Check sheet for the modelled part. Datum: model origin and axes. Units: mm. A direction names the side the tool comes from. Coordinates: 2 decimals unless noted, no trailing zeros. Loops run counter-clockwise (first coordinate to the right, second up) from the corner with the lowest first, then second, coordinate; pieces in that order, holes last.
```python
from build123d import *

# Parameters (mm, degrees)
F0_W     = 71.12
F0_H     = 71.12
F1_DEPTH = 43.18
F2_W     = 66.04
F2_H     = 66.04
F3_DEPTH = 40.64
F5_R     = 2.54
F4_W     = 71.12
F4_H     = 71.12
F4_W_2   = 3.81
F4_H_2   = 3.81
F6_DEPTH = 2.54
F7_R     = 2.53999


# Not quite as in the source:
# - a fillet or chamfer is up to 0.001 mm smaller than in the source, because OpenCascade refuses the exact size


with BuildPart() as f1:
    # F0 (on Top) → F1 (new body)
    with BuildSketch(Plane.XY):
        with Locations((35.56, 35.56)):
            Rectangle(F0_W, F0_H)
    extrude(amount=F1_DEPTH)

    # F2 (on face) → F3 (cut)
    with BuildSketch(Plane.XY.offset(43.18)):
        with Locations((35.56, 35.56)):
            Rectangle(F2_W, F2_H)
    extrude(amount=-F3_DEPTH, mode=Mode.SUBTRACT)

    # F5
    f5_edges = [f1.edges().sort_by_distance(p)[0] for p in [
        (71.12, 0, 21.59),
        (0, 0, 21.59),
        (0, 71.12, 21.59),
        (71.12, 71.12, 21.59),
    ]]
    fillet(f5_edges, radius=F5_R)

    # F4 (on face) → F6 (join)
    with BuildSketch(Plane(origin=(0, 0, 0), x_dir=(1, 0, 0), z_dir=(0, 0, -1))):
        Polygon((-3.81, -71.12), (0, -71.12), (0, -74.93), (74.93, -74.93), (74.93, 3.81), (-3.81, 3.81), align=None)
        with Locations((35.56, -35.56)):
            Rectangle(F4_W, F4_H, mode=Mode.SUBTRACT)
        with Locations((-1.905, -73.025)):
            Rectangle(F4_W_2, F4_H_2)
        with Locations((35.56, -35.56)):
            Rectangle(F4_W, F4_H)
    extrude(amount=F6_DEPTH)

    # F7 (radius 2.54 in the source; OpenCascade refuses exactly that, so slightly less here)
    f7_edges = [f1.edges().sort_by_distance(p)[0] for p in [
        (74.93, 35.56, -2.54),
        (35.56, -3.81, -2.54),
        (-3.81, 35.56, -2.54),
        (35.56, 74.93, -2.54),
        (-3.81, 74.93, -1.27),
        (74.93, 74.93, -1.27),
        (74.93, -3.81, -1.27),
        (-3.81, -3.81, -1.27),
    ]]
    fillet(f7_edges, radius=F7_R)


solid = f1.part
```
1) Scan lines: line 1 (Y direction, x = 55.5, z = 4.5); line 2 (Z direction, x = 4, y = 38). Record each from-to range of solid material in increasing order.
Answer sheet:
line 1: y = 0 to 2.54, 68.58 to 71.12
line 2: z = -2.54 to 2.54
2) Set-up check for faces 1 (the flat face through (35, 0, 21)), 2 (the cylindrical face through (0.724, 70.356, 21.892)), 3 (the flat face through (71.12, 35, 21)), 4 (the cylindrical face through (0.724, 0.764, 21.892)), 5 (the flat face through (2.54, 35, 23)): record each of +Z, -Z, +X, -X, +Y, -Y from which the full face is reachable in a straight line by a thin tool's end or side.
Answer sheet:
face 1: +Z, +X, -X, -Y
face 2: +Z, -X, +Y
face 3: +Z, +X, +Y, -Y
face 4: +Z, -X, -Y
face 5: +Z
3) Section check A-A on z = 13. Enter the section's corners in (x, y), plus the area to 3 significant figures.
Answer sheet:
outline: (0, 2.54) arc R2.54 ccw to (2.54, 0) - (68.58, 0) arc R2.54 ccw to (71.12, 2.54) - (71.12, 68.58) arc R2.54 ccw to (68.58, 71.12) - (2.54, 71.12) arc R2.54 ccw to (0, 68.58) - close; hole (2.54, 2.54) - (68.58, 2.54) - (68.58, 68.58) - (2.54, 68.58) - close
area: 691 mm2
4) Depth check by flat-ended pin: pin 1 (10 mm diameter, centred on x = 57, z = 22, fed in from +Y); pin 2 (3 mm diameter, centred on y = 7, z = 29, fed in from -X); pin 3 (12 mm diameter, centred on x = 44, z = 24, fed in from -Y). Enter the tip coordinate at first touch or a pass-through.
Answer sheet:
pin 1: stops at y = 71.12
pin 2: stops at x = 0
pin 3: stops at y = 0
5) Mould release check, pull along Y, two halves, no side actions. Record for faces 6 (the flat face through (0, 35, 21)), 7 (the cylindrical face through (36.076, 74.166, -1.816)), 8 (the flat face through (68.58, 35, 23)): +Y half, -Y half, draft (parallel to the pull), parting line (faces both ways), or undercut.
Answer sheet:
face 6: draft
face 7: +Y half
face 8: undercut
